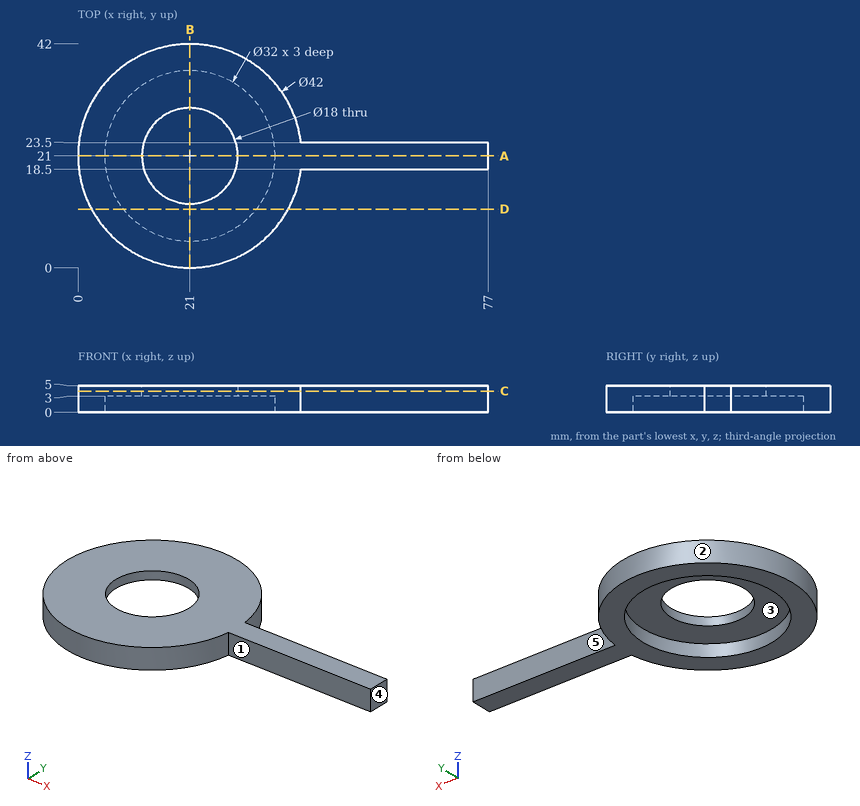
Source: three-view drawing plus pictorial views. Frame: mm from the lowest corner of the part. A direction names the side the tool comes from. Round coordinates to 2 decimals unless told otherwise and drop trailing zeros. Loops run counter-clockwise (first coordinate to the right, second up) from the corner with the lowest first, then second, coordinate; pieces in that order, holes last. Notation, with made-up numbers: M 68,87 L 77,87 A24 ccw 77,118 Z; hole C 16.25,17.25 d11. An arc over 180 degrees is marked long. Put each result on its own line as item: value. Start each with the question number.
(1) Section query D-D (y = 11). Return loops of the section in (x, z), then the cut area to 3 significant figures.
(2) Draft query along Y for the marked faces 1, 2 and 3. Return one class per face: +Y half, -Y half, draft (parallel to the pull), parting line (faces both ways), or undercut.
(3) Material intervals for line 1 along X through (y, z) = (21, 4.3); line 2 along Y through (x, z) = (21, 1.1); line 3 along X through (y, z) = (21, 1.1), sorted ascending. Write a range as [from, to].
(4) Section query A-A (y = 21). Return loops of the section in (x, z).
(5) Contact query for flat-ended pins moving along their axis: pin 1 Ø3 at (x, z) = (57.5, 1) entering from +Y; pin 2 Ø14.5 at (x, y) = (21, 21) entering from +Z; pin 3 Ø2.5 at (x, z) = (62, 3) entering from -Y; pin 4 Ø8 at (x, y) = (14, 12) entering from -Z. Output: stop coordinate, or through.
(6) Section query B-B (x = 21). Return loops of the section in (y, z), then the cut area to 3 significant figures.
(7) Section query C-C (z = 4). Return loops of the section in (x, y), then the cut area to 3 significant figures.
(8) Set-up query: the marked faces 4 and 5. Return all of +Z, -Z, +X, -X, +Y, -Y with unobstructed straight access to the full face (end or side cutting, diameter ignored); none if empty.
Findings below:
1. outline: M 2.53,0 L 8.51,0 L 8.51,3 L 33.49,3 L 33.49,0 L 39.47,0 L 39.47,5 L 2.53,5 Z
1. area: 110 mm2
2. face 1: -Y half
2. face 2: parting line
2. face 3: undercut
3. line 1: x = [0, 12], [30, 77]
3. line 2: y = [0, 5], [37, 42]
3. line 3: x = [0, 5], [37, 77]
4. outline: M 0,0 L 5,0 L 5,3 L 12,3 L 12,5 L 0,5 Z; M 30,3 L 37,3 L 37,0 L 77,0 L 77,5 L 30,5 Z
5. pin 1: stops at y = 23.5
5. pin 2: passes through
5. pin 3: stops at y = 18.5
5. pin 4: stops at z = 3
6. outline: M 0,0 L 5,0 L 5,3 L 12,3 L 12,5 L 0,5 Z; M 30,3 L 37,3 L 37,0 L 42,0 L 42,5 L 30,5 Z
6. area: 78.0 mm2
7. outline: M 41.85,18.5 L 77,18.5 L 77,23.5 L 41.85,23.5 A21 ccw long Z; hole C 21,21 d18
7. area: 1,310 mm2
8. face 4: +Z, -Z, +X, +Y, -Y
8. face 5: +Z, -Z, +X, +Y
